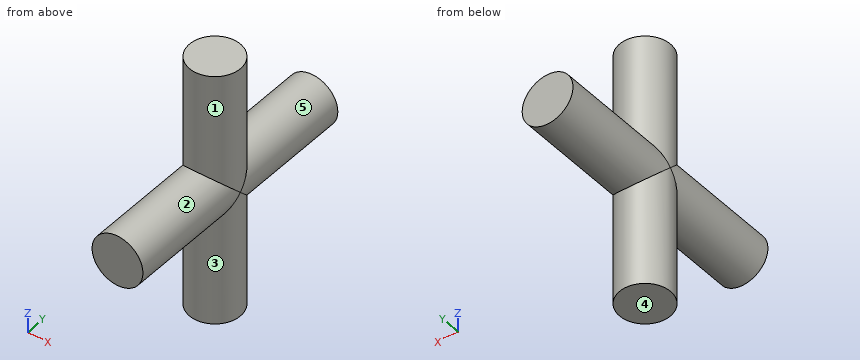
```python
from build123d import *

# Parameters (mm, degrees)
F0_R     = 2.5
F1_DEPTH = 12.5
F2_R     = 2.5
F3_DEPTH = 12.5


with BuildPart() as f1:
    # F0 (on Top) → F1 (new body, symmetric)
    with BuildSketch(Plane.XY):
        Circle(F0_R)
    extrude(amount=F1_DEPTH, both=True)

    # F2 (on Front) → F3 (join, symmetric)
    with BuildSketch(Plane.XZ):
        Circle(F2_R)
    extrude(amount=F3_DEPTH, both=True)


solid = f1.part
```
Geometry: final body of the model. Coordinates: model frame, mm. Face numbers are marked on the shaded views. A direction names the side the tool comes from. Round coordinates to 2 decimals unless told otherwise and drop trailing zeros. Loops run counter-clockwise (first coordinate to the right, second up) from the corner with the lowest first, then second, coordinate; pieces in that order, holes last. Notation, with made-up numbers: (52.5, -24) -> (93.5, -24) arc R30 ccw to (93.5, 15) -> close; hole circle Ø10 at (-4, 6.25). An arc over 180 degrees is marked (long way). Write each question's results on one line, items separated by ' | '.
Item 1: Cut plane C-C on y = 1.75. Return the cut outline in (x, z).
Answers below:
outline: (-1.79, -12.5) -> (1.79, -12.5) -> (1.79, -1.75) arc R2.5 ccw to (1.79, 1.75) -> (1.79, 12.5) -> (-1.79, 12.5) -> (-1.79, 1.75) arc R2.5 ccw to (-1.79, -1.75) -> close
Item 2: Cut plane B-B on z = 3.5. Return the cut outline in (x, y), and give its area (3 significant figures).
Answers below:
outline: circle Ø5 at (0, 0) | area: 19.6 mm²
Item 3: Set-up query: the marked faces 1, 2, 3, 4 and 5. Return all of +Z, -Z, +X, -X, +Y, -Y with unobstructed straight access to the full face (end or side cutting, diameter ignored); none if empty.
Answers below:
face 1: +Z | face 2: -Y | face 3: -Z | face 4: -Z, +X, -X, +Y, -Y | face 5: +Y
Item 4: Line query: probe 1 along Y at (x, z) = (0.2, -8.75); probe 2 along Z at (x, y) = (0.1, -10); probe 3 along Z at (x, y) = (-1.2, 5.25). Output: solid intervals per line, ascending. Write a range as [from, to].
Answers below:
probe 1: y = [-2.49, 2.49] | probe 2: z = [-2.5, 2.5] | probe 3: z = [-2.19, 2.19]
Item 5: Cut plane D-D on x = 1.4. Return the cut outline in (y, z).
Answers below:
outline: (-12.5, -2.07) -> (-2.07, -2.07) -> (-2.07, -12.5) -> (2.07, -12.5) -> (2.07, -2.07) -> (12.5, -2.07) -> (12.5, 2.07) -> (2.07, 2.07) -> (2.07, 12.5) -> (-2.07, 12.5) -> (-2.07, 2.07) -> (-12.5, 2.07) -> close
Item 6: Cut plane A-A on x = 0. Return the cut outline in (y, z), and give its area (3 significant figures).
Answers below:
outline: (-12.5, -2.5) -> (-2.5, -2.5) -> (-2.5, -12.5) -> (2.5, -12.5) -> (2.5, -2.5) -> (12.5, -2.5) -> (12.5, 2.5) -> (2.5, 2.5) -> (2.5, 12.5) -> (-2.5, 12.5) -> (-2.5, 2.5) -> (-12.5, 2.5) -> close | area: 225 mm²
